```python
from build123d import *


with BuildPart() as part:
    # Sketch1 → Revolve1 (revolve)
    with BuildSketch(Plane.XY):
        with BuildLine():
            Line((12.5, 0), (16, 0))
            Line((16, 0), (21.299800148, 19.568492854))
            ThreePointArc((21.299800148, 19.568492854), (23.444993074, 22.765026607), (27.09115838, 24))
            Line((27.09115838, 24), (38.716689233, 24))
            ThreePointArc((38.716689233, 24), (42.456896924, 22.69157185), (44.565840272, 19.336948809))
            Line((44.565840272, 19.336948809), (47.5, 6.5))
            Line((47.5, 6.5), (50, 6.5))
            Line((50, 6.5), (50, 51.5))
            Line((50, 51.5), (47.5, 51.5))
            Line((47.5, 51.5), (44.565840272, 38.663051191))
            ThreePointArc((44.565840272, 38.663051191), (42.456896924, 35.30842815), (38.716689233, 34))
            Line((38.716689233, 34), (27.09115838, 34))
            ThreePointArc((27.09115838, 34), (23.444993074, 35.234973393), (21.299800148, 38.431507146))
            Line((21.299800148, 38.431507146), (16, 58))
            Line((16, 58), (12.5, 58))
            Line((12.5, 58), (12.5, 0))
        make_face()
    revolve(axis=Axis((0, 0, 0), (0, 1, 0)))


solid = part.part
```
Input: part model. Units: mm. Frame: model coordinates. A direction names the side the tool comes from. Coordinates: 2 decimals unless noted, no trailing zeros. Write each loop counter-clockwise with the first axis right and the second up, starting at its lowest first coordinate (ties: lowest second). Pieces come first, ordered by that corner, then holes. Notation, with made-up numbers: M 34,15 L 81,15 A5 cw 81,22 Z; hole C -18.75,27 d3. An arc over 180 degrees is marked long. Use one line per item in the form item = value.
Q1. Set-up query: faces 1 (the face through (44.2, 51.5, 18.3)), 2 (the face through (10, 0, 8)), 3 (the face through (-44.2, 6.5, 18.3)). Return all of +Z, -Z, +X, -X, +Y, -Y with unobstructed straight access to the full face (end or side cutting, diameter ignored); none if empty.
Answer below:
face_1 = +Y
face_2 = +Z, -Z, +X, -X, -Y
face_3 = -Y
Q2. Section C-C (y = 50). Return loops of the section in (x, z).
Answer below:
outline = C 0,0 d100; C 0,0 d36.33; hole C 0,0 d94.31; hole C 0,0 d25
Q3. First-contact query: pin 1 (1.5 mm diameter, centred on x = -17.5, y = 6, fed in from +Z); pin 2 (6 mm diameter, centred on y = 37.5, z = 4, fed in from -X); pin 3 (4 mm diameter, centred on x = 31.5, z = -25, fed in from -Y). Flat tips, straight axial feed; report the tip coordinate or a pass-through.
Answer below:
pin_1 = 47.04
pin_2 = -49.99
pin_3 = 22.87
Q4. Section D-D (y = 29.5). Return loops of the section in (x, z).
Answer below:
outline = C 0,0 d100; hole C 0,0 d25
Q5. Draft query along X for faces 4 (the face through (47.69, 29.32, -15.02)), 5 (the face through (-10, 58, 8)), 6 (the face through (-35.479, 39.286, 27.204)). Return one class per face: released by +X, released by -X, zero draft, split by the parting line, or undercut.
Answer below:
face_4 = split by the parting line
face_5 = zero draft
face_6 = undercut
Q6. Material intervals for probe 1 along Z at (x, y) = (0, 33); probe 2 along X at (y, z) = (34.5, 0); probe 3 along X at (y, z) = (44.5, -6.5), sorted ascending. Write a range as from..to.
Answer below:
probe_1 = -50..-12.5, 12.5..50
probe_2 = -50..-41.11, -24.69..-12.5, 12.5..24.69, 41.11..50
probe_3 = -49.58..-45.44, -18.55..-10.68, 10.68..18.55, 45.44..49.58
